The figure shows three views and two pictorial views of one solid part (mm, origin at its lowest corner). Answer the questions. A direction names the side the tool comes from. Give positions to 0.01 mm unless a question says otherwise; leave off trailing zeros. Write each loop counter-clockwise with the first axis right and the second up, starting at its lowest first coordinate (ties: lowest second). Pieces come first, ordered by that corner, then holes. Notation, with made-up numbers: (55.25, -6.75) - (103.25, -6.75) arc R15 cw to (103.25, 1.25) - close; hole circle Ø9 at (-37, 68). An arc over 180 degrees is marked (long way). Answer as CSV lines item,"result". Start each with the question number.
(1) Straight lines are drawn through the part: probe 1 along Z at (x, y) = (20, 54.15); probe 2 along X at (y, z) = (54, 8); probe 3 along Y at (x, z) = (88, 9). For each, find the intervals that lie inside material, in ascending order.
(2) Find section B-B (y = 46). Write down the section's boundary in (x, z).
(3) Find section C-C (x = 20). Write down the section's boundary in (y, z), then the cut area to 4 significant figures.
(4) Each of these flat-tipped pins is pushed along its axis until it touches: pin 1 Ø4 at (x, y) = (74.5, 15.5) entering from -Z; pin 2 Ø8 at (x, z) = (20, 8) entering from -Y; pin 3 Ø5.5 at (x, z) = (55.5, 28) entering from +Y. Where does it stop, or does it pass through?
(5) Find section A-A (z = 18.25). Write down the section's boundary in (x, y), then the cut area to 3 significant figures.
(6) For the marked faces 1 and 2, determine the directions among +Z, -Z, +X, -X, +Y, -Y from which every point of the face is accessible in a straight line to the end or side of a thin tool.
(7) Find section D-D (z = 8). Write down the section's boundary in (x, y), then the cut area to 3 significant figures.
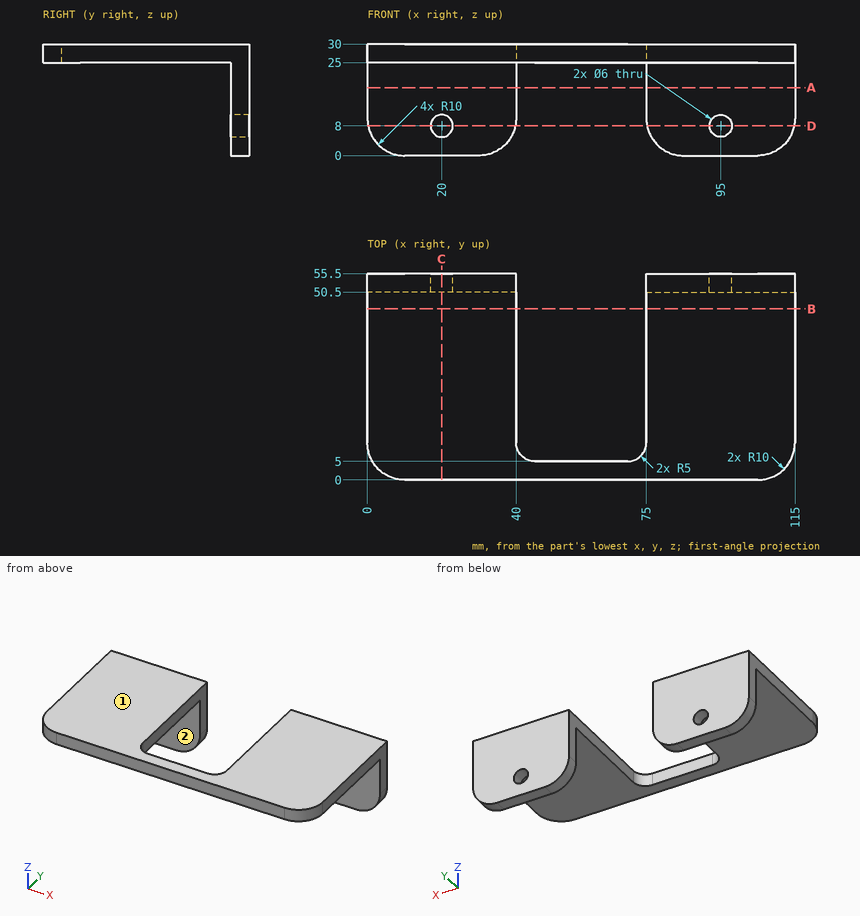
Result set:
1,probe 1,"0 to 5, 11 to 30"
1,probe 2,"0.2 to 17, 23 to 39.8, 75.2 to 92, 98 to 114.8"
1,probe 3,"50.5 to 55.5"
2,outline,"(0, 25) - (40, 25) - (40, 30) - (0, 30) - close; (75, 25) - (115, 25) - (115, 30) - (75, 30) - close"
3,outline,"(0, 25) - (50.5, 25) - (50.5, 11) - (55.5, 11) - (55.5, 30) - (0, 30) - close; (50.5, 0) - (55.5, 0) - (55.5, 5) - (50.5, 5) - close"
3,area,"372.5 mm^2"
4,pin 1,"z = 25"
4,pin 2,"y = 50.5"
4,pin 3,"y = 5"
5,outline,"(0, 50.5) - (40, 50.5) - (40, 55.5) - (0, 55.5) - close; (75, 50.5) - (115, 50.5) - (115, 55.5) - (75, 55.5) - close"
5,area,"400 mm^2"
6,face 1,"+Z, +X, -X, +Y, -Y"
6,face 2,"-Z, +X, -X, -Y"
7,outline,"(0.2, 50.5) - (17, 50.5) - (17, 55.5) - (0.2, 55.5) - close; (23, 50.5) - (39.8, 50.5) - (39.8, 55.5) - (23, 55.5) - close; (75.2, 50.5) - (92, 50.5) - (92, 55.5) - (75.2, 55.5) - close; (98, 50.5) - (114.8, 50.5) - (114.8, 55.5) - (98, 55.5) - close"
7,area,"336 mm^2"
